```python
from build123d import *

# Parameters (mm, degrees)
SKETCH1_R           = 3
SKETCH1_W           = 25
SKETCH1_H           = 6
BOSS_EXTRUDE1_DEPTH = 6


with BuildPart() as part:
    # Sketch1 → Boss-Extrude1 (new body)
    with BuildSketch(Plane(origin=(0, 0, 0), x_dir=(1, 0, 0), z_dir=(0, 1, 0))):
        with BuildLine():
            Line((-18.981997388, -27.5), (21.018002612, -27.5))
            Line((21.018002612, -27.5), (21.018002612, 23.5))
            ThreePointArc((21.018002612, 23.5), (18.089070424, 30.571067812), (11.018002612, 33.5))
            Line((11.018002612, 33.5), (-8.981997388, 33.5))
            ThreePointArc((-8.981997388, 33.5), (-16.053065199, 30.571067812), (-18.981997388, 23.5))
            Line((-18.981997388, 23.5), (-18.981997388, -27.5))
        make_face()
        with Locations((1.018002612, 18.5)):
            Circle(SKETCH1_R, mode=Mode.SUBTRACT)
        with Locations((1.018002612, -19.214324507)):
            Rectangle(SKETCH1_W, SKETCH1_H, mode=Mode.SUBTRACT)
    extrude(amount=BOSS_EXTRUDE1_DEPTH)


solid = part.part
```
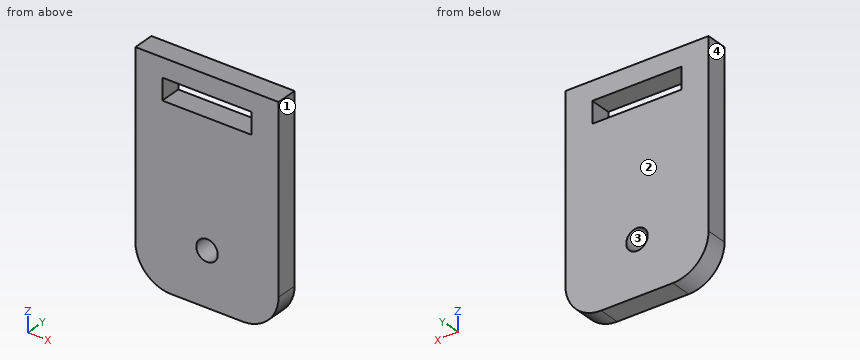
Read the model definition and answer for the solid it produces. Units are mm, in the model's axes. Face numbers are marked on the shaded views. Give positions to 0.01 mm unless a question says otherwise; leave off trailing zeros. Order: outer loops, then holes, each group sorted by start corner. A loop starts at its lowest first (then second) coordinate and runs counter-clockwise, first axis right, second up.
(1) Straight lines are drawn through the part: L1, parallel to X at y = 2.6, z = -18.5; L2, parallel to Z at x = 10, y = 4.1; L3, parallel to X at y = 2.8, z = 18. For each, find the intervals that lie inside material, in ascending order.
(2) Find section D-D (z = -26.5). Give the vertices of the cut face in (x, y).
(3) For a pull along X with two mould halves and no side action, classify the marked faces 1, 2, 3 and 4 as released by +X, released by -X, zero draft, split by the parting line, or undercut.
(4) Find section B-B (x = 8.5). Give the vertices of the cut face in (y, z).
(5) Find section A-A (z = 18.5). Give the vertices of the cut face in (x, y).
(6) Find section C-C (y = 3). Give the vertices of the cut face in (x, z), plus the area to 3 significant figures.
Result sheet:
1. L1: x = -18.98 to -1.98, 4.02 to 21.02
1. L2: z = -33.5 to 16.21, 22.21 to 27.5
1. L3: x = -18.98 to -11.48, 13.52 to 21.02
2. outline: (-18.52, 0) - (20.56, 0) - (20.56, 6) - (-18.52, 6) - close
3. face 1: released by +X
3. face 2: zero draft
3. face 3: undercut
3. face 4: released by -X
4. outline: (0, -33.5) - (6, -33.5) - (6, 16.21) - (0, 16.21) - close; (0, 22.21) - (6, 22.21) - (6, 27.5) - (0, 27.5) - close
5. outline: (-18.98, 0) - (-11.48, 0) - (-11.48, 6) - (-18.98, 6) - close; (13.52, 0) - (21.02, 0) - (21.02, 6) - (13.52, 6) - close
6. outline: (-18.98, -23.5) arc R10 ccw to (-8.98, -33.5) - (11.02, -33.5) arc R10 ccw to (21.02, -23.5) - (21.02, 27.5) - (-18.98, 27.5) - close; hole (-11.48, 16.21) - (13.52, 16.21) - (13.52, 22.21) - (-11.48, 22.21) - close; hole circle Ø6 at (1.02, -18.5)
6. area: 2,220 mm2
